Study the drawing (mm; zero at the part's minimum x, y, z) and answer. Round coordinates to 2 decimals unless told otherwise and drop trailing zeros. Write each loop counter-clockwise with the first axis right and the second up, starting at its lowest first coordinate (ties: lowest second). Pieces come first, ordered by that corner, then holes. Notation, with made-up numbers: (-22, 47) - (26, 47) arc R19 cw to (26, 77) - close; hole circle Ø8 at (45, 70.25). An arc over 180 degrees is marked (long way). Use one line per item in the form item = value. Start each with the question number.
1) Consider line 1 along Y through (x, z) = (33, 8.5); line 2 along Z through (x, y) = (20.5, 0.5); line 3 along X through (y, z) = (2.25, 16). Determine where each line is inside the solid, lowest interval first. Write a range as from..to.
2) The part is cut by section C-C, the plane x = 42. Give the vertices of the cut face in (y, z).
3) The part is cut by section A-A, the plane y = 3.25. Give the vertices of the cut face in (x, z), plus the area to 3 significant figures.
4) Each of these flat-tipped pins is pushed along its axis until it touches: pin 1 (19 mm diameter, centred on x = 51.5, z = 22, fed in from -Y); pin 2 (1.5 mm diameter, centred on y = 1, z = 44.5, fed in from -X); pin 3 (6 mm diameter, centred on x = 23.5, z = 35, fed in from -Y). Where does it stop, or does it pass through?
5) The part is cut by section B-B, the plane z = 36. Give the vertices of the cut face in (x, y), plus the area to 3 significant figures.
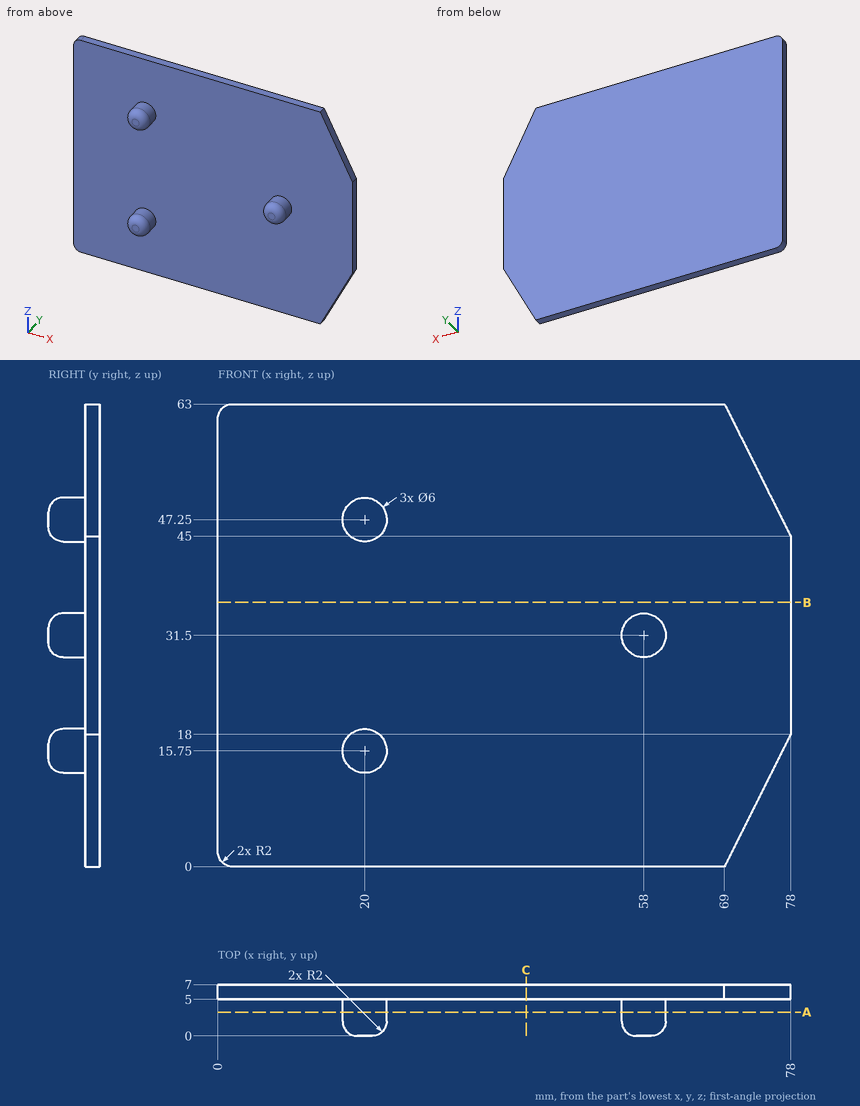
Geometry results:
q1.line_1 = 5..7
q1.line_2 = 13.48..18.02, 44.98..49.52
q1.line_3 = 17.01..22.99
q2.outline = (5, 0) - (7, 0) - (7, 63) - (5, 63) - close
q3.outline = circle Ø6 at (20, 15.75); circle Ø6 at (20, 47.25); circle Ø6 at (58, 31.5)
q3.area = 84.8 mm2
q4.pin_1 = 0.27
q4.pin_2 = 18
q4.pin_3 = 5
q5.outline = (0, 5) - (78, 5) - (78, 7) - (0, 7) - close
q5.area = 156 mm2
